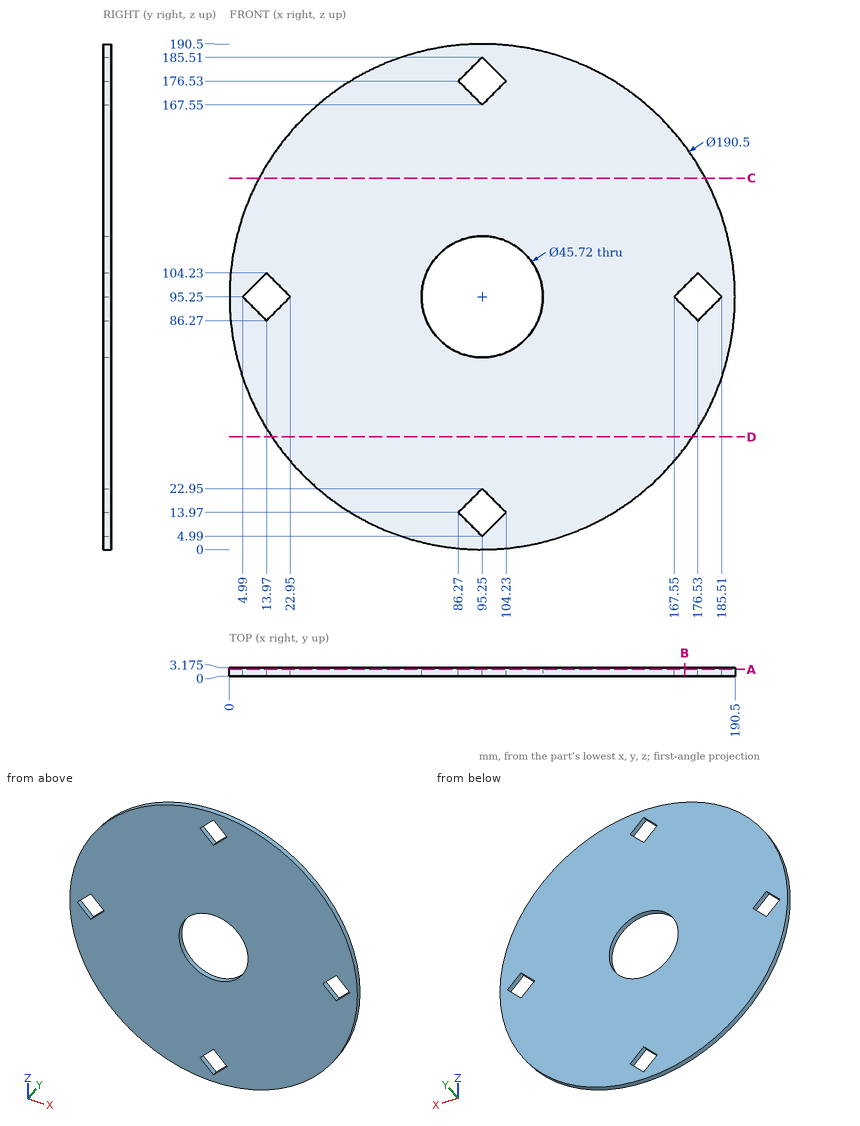
Input: dimensioned drawing with shaded views. Units: mm. Origin: part minimum x, y, z. Coordinates: 2 decimals unless noted, no trailing zeros. Order: outer loops, then holes, each group sorted by start corner. A loop starts at its lowest first (then second) coordinate and runs counter-clockwise, first axis right, second up.
1. Cut plane D-D, the plane z = 42.5. Return loops of the section in (x, y) (1 decimal).
Checked values:
outline: (15.9, 0) - (174.6, 0) - (174.6, 3.2) - (15.9, 3.2) - close
2. Cut plane B-B, the plane x = 171.5. Return loops of the section in (y, z) (1 decimal).
Checked values:
outline: (0, 38.2) - (3.2, 38.2) - (3.2, 91.3) - (0, 91.3) - close; (0, 99.2) - (3.2, 99.2) - (3.2, 152.3) - (0, 152.3) - close
3. Contact query for flat-ended pins moving along their axis: P1, Ø1, axis at x = 47.5, y = 1, coming from the +Z side (1 decimal); P2, Ø1, axis at x = 27.5, y = 0.5, coming from the +Z side; P3, Ø2, axis at x = 103.5, z = 114, coming from the -Y side. Output: stop coordinate, or through.
Checked values:
P1: stops at z = 178
P2: stops at z = 162.7
P3: passes through
4. Cut plane A-A, the plane y = 2.45. Return loops of the section in (x, z).
Checked values:
outline: circle Ø190.5 at (95.25, 95.25); hole (4.99, 95.25) - (13.97, 86.27) - (22.95, 95.25) - (13.97, 104.23) - close; hole circle Ø45.72 at (95.25, 95.25); hole (86.27, 13.97) - (95.25, 4.99) - (104.23, 13.97) - (95.25, 22.95) - close; hole (86.27, 176.53) - (95.25, 167.55) - (104.23, 176.53) - (95.25, 185.51) - close; hole (167.55, 95.25) - (176.53, 86.27) - (185.51, 95.25) - (176.53, 104.23) - close
5. Cut plane C-C, the plane z = 140. Return loops of the section in (x, y) (1 decimal), plus the area to 3 significant figures.
Checked values:
outline: (11.2, 0) - (179.3, 0) - (179.3, 3.2) - (11.2, 3.2) - close
area: 534 mm2
6. Ray query, line 1 along Z through (x, y) = (95.25, 1.9); line 2 along Z through (x, y) = (99, 1.9) (1 decimal); line 3 along Z through (x, y) = (12, 0.6). Return the intervals inside material, ascending.
Checked values:
line 1: z = 0 to 4.99, 22.95 to 72.39, 118.11 to 167.55, 185.51 to 190.5
line 2: z = 0.1 to 8.7, 19.2 to 72.7, 117.8 to 171.3, 181.8 to 190.4
line 3: z = 48.97 to 88.24, 102.26 to 141.53
